The listing builds one solid part. Answer for the finished solid, in the listing's coordinates (mm). A direction names the side the tool comes from. Coordinates: 2 decimals unless noted, no trailing zeros. Order: outer loops, then holes, each group sorted by start corner. A loop starts at its lowest first (then second) coordinate and runs counter-clockwise, first axis right, second up. Notation, with made-up numbers: (-27, -25) -> (-2, -25) arc R22 ccw to (-2, 13) -> close; hole circle Ø6 at (68, 80). An arc over 180 degrees is marked (long way). Return JSON: item names as keys, results as strings.
```python
from build123d import *

# Parameters (mm, degrees)
SKETCH1_W                      = 80
SKETCH1_H                      = 40
BASE_FLANGE1_DEPTH             = 2
EDGE_FLANGE1_STRIP_W           = 12
EDGE_FLANGE1_STRIP_H           = 2
EDGE_FLANGE1_STRIP_CUT_DEPTH   = 40
EDGE_FLANGE1_STRIP_2_W         = 12
EDGE_FLANGE1_STRIP_2_H         = 2
EDGE_FLANGE1_STRIP_CUT_2_DEPTH = 40
EDGE_FLANGE1_DEPTH             = 40
EDGE_FLANGE1_BEND_DEPTH        = 40
SKETCH12_R                     = 6.5
SKETCH12_R_2                   = 2.5
CUT_EXTRUDE1_DEPTH             = 10
SKETCH13_W                     = 6
SKETCH13_H                     = 40
CUT_EXTRUDE2_DEPTH             = 25


# Sheet-metal steps are written as plain solids
with BuildPart() as part:
    # Sketch1 → Base-Flange1 (new body)
    with BuildSketch(Plane(origin=(0, 0, 0), x_dir=(1, 0, 0), z_dir=(0, 1, 0))):
        Rectangle(SKETCH1_W, SKETCH1_H)
    extrude(amount=-BASE_FLANGE1_DEPTH)

    # Edge-Flange1 strip (across the edge) → Edge-Flange1 strip cut (cut)
    with BuildSketch(Plane(origin=(-40, 0, -20), x_dir=(1, 0, 0), z_dir=(0, 0, 1))):
        with Locations((-2, -1)):
            Rectangle(EDGE_FLANGE1_STRIP_W, EDGE_FLANGE1_STRIP_H)
    extrude(amount=EDGE_FLANGE1_STRIP_CUT_DEPTH, mode=Mode.SUBTRACT)

    # Edge-Flange1 strip 2 (across the edge) → Edge-Flange1 strip cut 2 (cut)
    with BuildSketch(Plane(origin=(40, 0, 20), x_dir=(-1, 0, 0), z_dir=(0, 0, -1))):
        with Locations((-2, -1)):
            Rectangle(EDGE_FLANGE1_STRIP_2_W, EDGE_FLANGE1_STRIP_2_H)
    extrude(amount=EDGE_FLANGE1_STRIP_CUT_2_DEPTH, mode=Mode.SUBTRACT)

    # Edge-Flange1 section (across the edge) → Edge-Flange1 (add)
    with BuildSketch(Plane(origin=(-40, 0, -20), x_dir=(1, 0, 0), z_dir=(0, 0, 1))):
        with BuildLine():
            Line((0, 2), (0, 33))
            Line((0, 33), (2, 33))
            Line((2, 33), (2, 2))
            ThreePointArc((2, 2), (2.585786438, 0.585786438), (4, 0))
            Line((4, 0), (4, -2))
            ThreePointArc((4, -2), (1.171572875, -0.828427125), (0, 2))
        make_face()
    extrude(amount=EDGE_FLANGE1_DEPTH)

    # Edge-Flange1 section 2 (across the edge) → Edge-Flange1 bend (add)
    with BuildSketch(Plane(origin=(40, 0, 20), x_dir=(-1, 0, 0), z_dir=(0, 0, -1))):
        with BuildLine():
            Line((0, 2), (0, 33))
            Line((0, 33), (2, 33))
            Line((2, 33), (2, 2))
            ThreePointArc((2, 2), (2.585786438, 0.585786438), (4, 0))
            Line((4, 0), (4, -2))
            ThreePointArc((4, -2), (1.171572875, -0.828427125), (0, 2))
        make_face()
    extrude(amount=EDGE_FLANGE1_BEND_DEPTH)

    # Sketch12 → Cut-Extrude1 (cut)
    with BuildSketch(Plane(origin=(40, 0, 0), x_dir=(0, 0, -1), z_dir=(1, 0, 0))):
        with Locations(Location((0, 18, 0), (0, 0, 90))):
            Circle(SKETCH12_R)
        with Locations(Location((-11, 18, 0), (0, 0, 90))):
            Circle(SKETCH12_R_2)
        with Locations(Location((11, 18, 0), (0, 0, 270))):
            Circle(SKETCH12_R_2)
    extrude(amount=-CUT_EXTRUDE1_DEPTH, mode=Mode.SUBTRACT)

    # Sketch13 → Cut-Extrude2 (cut)
    with BuildSketch(Plane.ZY.offset(40)):
        with Locations((9, -2)):
            Rectangle(SKETCH13_W, SKETCH13_H)
        with Locations((-9, -2)):
            Rectangle(SKETCH13_W, SKETCH13_H)
    extrude(amount=-CUT_EXTRUDE2_DEPTH, mode=Mode.SUBTRACT)


solid = part.part
```
Item 1: Determine the mould class of faces 6 (the flat face through (-38, 18, 0)), 7 (the flat face through (0, -1, -20)), 8 (the cylindrical face through (39, 20, -9.5)) for opening direction Z: pulls with the +Z half, pulls with the -Z half, needs draft (parallel to the pull), parting line crosses it, or undercut.
Answer list:
{"face 6": "needs draft", "face 7": "pulls with the -Z half", "face 8": "undercut"}
Item 2: Which of the six approach directions +Z, -Z, +X, -X, +Y, -Y give full straight-line access (tool end or side, diameter ignored) to faces 1 (the cylindrical face through (-38.797, -0.859, 15.944)), 2 (the cylindrical face through (-37.43, 0.6, -0.08)), 3 (the flat face through (-39, 18, -9)), 4 (the flat face through (-15, -1, 9)), 5 (the cylindrical face through (39.014, 11.506, 0.286))?
Answer list:
{"face 1": "+Z, -Z, -X, -Y", "face 2": "+Z, -Z, +Y", "face 3": "-X, -Y", "face 4": "-X, +Y, -Y", "face 5": "+X"}
Item 3: The part is cut by section D-D on x = -28. Determine the outline of the cut face in (y, z).
Answer list:
{"outline": "(-2, -20) -> (0, -20) -> (0, -12) -> (-2, -12) -> close; (-2, -6) -> (0, -6) -> (0, 6) -> (-2, 6) -> close; (-2, 12) -> (0, 12) -> (0, 20) -> (-2, 20) -> close"}
Item 4: Find the intervals of material crossed by probe 1 along Z at (x, y) = (38.85, 18); probe 2 along X at (y, z) = (10, 1); probe 3 along X at (y, z) = (14.5, 8), in increasing order.
Answer list:
{"probe 1": "-20 to -13.5, -8.5 to -6.5, 6.5 to 8.5, 13.5 to 20", "probe 2": "-40 to -38, 38 to 40", "probe 3": "38 to 40"}
Item 5: The part is cut by section B-B on z = -9.5. Determine the outline of the cut face in (x, y).
Answer list:
{"outline": "(-40, 18) -> (-38, 18) -> (-38, 33) -> (-40, 33) -> close; (-15, -2) -> (36, -2) arc R4 ccw to (40, 2) -> (40, 16) -> (38, 16) -> (38, 2) arc R2 cw to (36, 0) -> (-15, 0) -> close; (38, 20) -> (40, 20) -> (40, 33) -> (38, 33) -> close"}
Item 6: The part is cut by section C-C on y = 26.5. Determine the outline of the cut face in (x, z).
Answer list:
{"outline": "(-40, -20) -> (-38, -20) -> (-38, 20) -> (-40, 20) -> close; (38, -20) -> (40, -20) -> (40, 20) -> (38, 20) -> close"}
Item 7: The part is cut by section A-A on y = 9. Determine the outline of the cut face in (x, z), plus the area to 3 significant figures.
Answer list:
{"outline": "(-40, -20) -> (-38, -20) -> (-38, -12) -> (-40, -12) -> close; (-40, -6) -> (-38, -6) -> (-38, 6) -> (-40, 6) -> close; (-40, 12) -> (-38, 12) -> (-38, 20) -> (-40, 20) -> close; (38, -20) -> (40, -20) -> (40, 20) -> (38, 20) -> close", "area": "136 mm2"}
Item 8: Flat-ended cylindrical pins translate along their axes: pin 1 (4 mm diameter, centred on y = 18, z = -11, fed in from +X); pin 2 (20 mm diameter, centred on x = -16, z = 9.5, fed in from +Y); pin 3 (0.6 mm diameter, centred on x = -39.5, z = 8, fed in from -Y); pin 4 (10 mm diameter, centred on x = -28, y = 8, fed in from +Z). Find the tip coordinate at first contact, or state that the pin passes through.
Answer list:
{"pin 1": "x = -38", "pin 2": "y = 0", "pin 3": "y = 18", "pin 4": "through"}
